Autodesk Inventor part; units mm, degrees
ref_plane "YZ Plane" through (0, 0, 0) normal (1, 0, 0) x (0, 1, 0)
ref_plane "XZ Plane" through (0, 0, 0) normal (0, 1, 0) x (-1, 0, 0)
ref_plane "XY Plane" through (0, 0, 0) normal (0, 0, 1) x (1, 0, 0)
sketch "Sketch1" plane through (0, 0, 0) normal (0, 0, 1) x (1, 0, 0)
  line L0 (0, 0) -> (53, 0)
  line L1 (53, 0) -> (53, 30)
  line L2 (53, 30) -> (0, 30)
  line L3 (0, 30) -> (0, 0)
  point P0 (2.5, 2.5)
  point P1 (50.5, 2.5)
  point P2 (50.5, 27.5)
  dimension "d0" = 53
  dimension "d1" = 30
extrude "Extrusion1" add sketch "Sketch1" along normal blind 3
hole "Hole1" at (2.5, 2.5, 0) at (50.5, 2.5, 0) at (50.5, 27.5, 0) direction (0, 0, 1) diameter 3 end through all
sketch "Sketch2" plane through (0, 0, 3) normal (0, 0, 1) x (1, 0, 0)
  line L0 (53, 0) -> (53, 30)
  line L1 (53, 30) -> (48, 30)
  line L2 (53, 30) -> (0, 30)
  line L3 (48, 30) -> (0, 25.3519)
  line L4 (0, 30) -> (0, 0)
  line L5 (0, 30) -> (48, 30)
  dimension "d11" = 5
extrude "Extrusion2" cut sketch "Sketch2" against normal through all
properties part number "head-sideplate" material "Aluminum 6061"
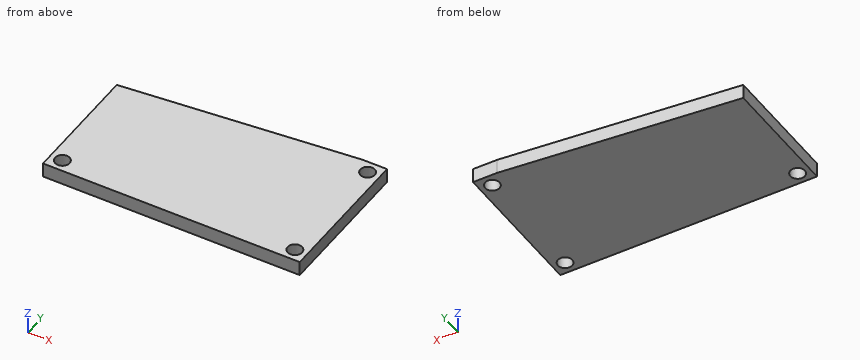
CAD build for the part. Positions are in the model's coordinates, mm. Round coordinates to 2 decimals unless told otherwise and drop trailing zeros. Write each loop counter-clockwise with the first axis right and the second up, starting at its lowest first coordinate (ties: lowest second). Pieces come first, ordered by that corner, then holes. Notation, with made-up numbers: (2.25, 37.25) -> (10.25, 37.25) arc R4 cw to (10.25, 41.25) -> close; hole circle Ø6 at (88.25, 0.5). An arc over 180 degrees is marked (long way). Answer in a Markdown table with one row per item. Add a question column.
Item 1: Saw through at A-A, the plane y = 2.5. Write the cut outline in (x, z).
Item 2: Drop a flat-ended pin along its axis: pin 1 Ø2.5 at (x, y) = (2.5, 2.5) entering from +Z. Give the stop position or say it passes through.
Item 3: Drill centre lines: line 1 (Y direction, x = 50.5, z = 0.8); line 2 (X direction, y = 2.5, z = 1.55); line 3 (Y direction, x = 2.5, z = 1.65). Where is each one in solid material? Low to high. Write a range as from..to.
Item 4: Saw through at D-D, the plane y = 27.5. Write the cut outline in (x, z), then the cut area to 3 significant figures.
Item 5: Saw through at C-C, the plane x = 2.5. Write the cut outline in (y, z), then the cut area to 3 significant figures.
Item 6: Saw through at B-B, the plane z = 2.45. Write the cut outline in (x, y), then the cut area to 3 significant figures.
Findings below:
| question | item | result |
|---|---|---|
| 1 | outline | (0, 0) -> (1, 0) -> (1, 3) -> (0, 3) -> close; (4, 0) -> (49, 0) -> (49, 3) -> (4, 3) -> close; (52, 0) -> (53, 0) -> (53, 3) -> (52, 3) -> close |
| 2 | pin 1 | passes through |
| 3 | line 1 | y = 0..1, 4..26, 29..30 |
| 3 | line 2 | x = 0..1, 4..49, 52..53 |
| 3 | line 3 | y = 0..1, 4..25.59 |
| 4 | outline | (22.18, 0) -> (49, 0) -> (49, 3) -> (22.18, 3) -> close; (52, 0) -> (53, 0) -> (53, 3) -> (52, 3) -> close |
| 4 | area | 83.5 mm^2 |
| 5 | outline | (0, 0) -> (1, 0) -> (1, 3) -> (0, 3) -> close; (4, 0) -> (25.59, 0) -> (25.59, 3) -> (4, 3) -> close |
| 5 | area | 67.8 mm^2 |
| 6 | outline | (0, 0) -> (53, 0) -> (53, 30) -> (48, 30) -> (0, 25.35) -> close; hole circle Ø3 at (2.5, 2.5); hole circle Ø3 at (50.5, 2.5); hole circle Ø3 at (50.5, 27.5) |
| 6 | area | 1,460 mm^2 |
